```python
from build123d import *

# Parameters (mm, degrees)
F1_DEPTH = 11.0582
F2_SCALE = 0.3


with BuildPart() as f1:
    # F0 (on Front) → F1 (new body)
    with BuildSketch(Plane.XZ):
        Polygon((0.806323, 147.5619096), (-16.5301676, 29.8349162), (-49.993677, 60.879355), (-34.673032, 17.3364906), (-113.2920772, 8.063484), (-32.657161, -10.8857288), (-59.2666836, -42.736516), (-16.9333418, -25.8031742), (-2.54e-05, -147.5619096), (16.5301422, -24.9968258), (60.4761808, -42.3333418), (34.2698324, -10.0793804), (113.2920518, 8.4666582), (35.479355, 17.3364906), (49.9936262, 60.4761808), (16.9333164, 27.8190452), align=None)
    extrude(amount=F1_DEPTH)


with BuildPart() as f1_1:
    # F2: moved
    add(f1.part.scale(F2_SCALE).moved(Location((0.5644261, -7.74074, 103.29333672))))


with BuildPart() as f1_2:
    # F3: moved
    add(f1_1.part.moved(Location((59.91897, 0, -43.45396))))


solid = f1_2.part
```
Here's how the part is built. I have some questions about the finished solid (model axes, mm). A direction names the side the tool comes from. Give positions to 0.01 mm unless a question says otherwise; leave off trailing zeros. Loops run counter-clockwise (first coordinate to the right, second up) from the corner with the lowest first, then second, coordinate; pieces in that order, holes last. Notation, with made-up numbers: (55.5, 9) -> (94.5, 9) arc R12 cw to (94.5, 20) -> close; hole circle Ø1 at (43.25, 72.5). An arc over 180 degrees is marked (long way). Use one line per item in the form item = value. Start each with the question number.
1) Imagine slicing it at A-A (z = 74). Please give me the cut outline in (x, y), then the cut area to 3 significant figures.
2) Which directions (+Z, -Z, +X, -X, +Y, -Y) give clear straight access to the entire face, cutting with the end or side of a thin tool? Please do faces 5 (the face through (71.942, -9.376, 49.776)), 6 (the face through (74.75, -9.38, 51.91)), 7 (the face through (60, -7.741, 60)), 8 (the face through (38.45, -9.38, 63.67)), 9 (the face through (50.575, -9.376, 73.381)).
3) Imagine slicing it at B-B (x = 46.5). Please give me the cut outline in (y, z), then the cut area to 3 significant figures.
4) Imagine slicing it at C-C (y = -9.25). Please give me the cut outline in (x, z), then the cut area to 3 significant figures.
5) Imagine slicing it at D-D (x = 31.5). Please give me the cut outline in (y, z).
6) Thinking about a two-plate mould opening in X: for faces 1 (the face through (47.751, -9.376, 71.663)), 2 (the face through (48.96, -9.38, 49.52)), 3 (the face through (70.59, -9.38, 73.15)), 4 (the face through (82.96, -9.38, 63.69)), which applies, +X half, -X half, draft (parallel to the pull), parting line (faces both ways), or undercut?
7) Please list where these lines run through material, in increasing order: line 1 along X through (y, z) = (-10, 73); line 2 along X through (y, z) = (-8.3, 76.5); line 3 along Z through (x, y) = (77, -9.55).
Check values:
q1.outline = (46.93, -11.06) -> (49.91, -11.06) -> (49.91, -7.74) -> (46.93, -7.74) -> close; (56.29, -11.06) -> (64.78, -11.06) -> (64.78, -7.74) -> (56.29, -7.74) -> close; (71.45, -11.06) -> (74.14, -11.06) -> (74.14, -7.74) -> (71.45, -7.74) -> close
q1.area = 47.0 mm^2
q2.face_5 = -Z, +Y, -Y
q2.face_6 = +X, +Y, -Y
q2.face_7 = +Z, -Z, +X, -X, +Y
q2.face_8 = -X, +Y, -Y
q2.face_9 = +Z, +Y, -Y
q3.outline = (-11.06, 48.54) -> (-7.74, 48.54) -> (-7.74, 51.56) -> (-11.06, 51.56) -> close; (-11.06, 57.56) -> (-7.74, 57.56) -> (-7.74, 64.62) -> (-11.06, 64.62) -> close; (-11.06, 75.22) -> (-7.74, 75.22) -> (-7.74, 77.16) -> (-11.06, 77.16) -> close
q3.area = 39.9 mm^2
q4.outline = (26.5, 62.26) -> (50.69, 56.57) -> (42.7, 47.02) -> (55.4, 52.1) -> (60.48, 15.57) -> (65.44, 52.34) -> (78.63, 47.14) -> (70.76, 56.82) -> (94.47, 62.38) -> (71.13, 65.04) -> (75.48, 77.98) -> (65.56, 68.19) -> (60.73, 104.11) -> (55.52, 68.79) -> (45.49, 78.1) -> (50.08, 65.04) -> close
q4.area = 1,020 mm^2
q5.outline = (-11.06, 61.08) -> (-7.74, 61.08) -> (-7.74, 62.85) -> (-11.06, 62.85) -> close
q6.face_1 = -X half
q6.face_2 = undercut
q6.face_3 = undercut
q6.face_4 = +X half
q7.line_1 = 47.28 to 50.99, 56.14 to 64.91, 70.44 to 73.81
q7.line_2 = 46.05 to 47.21, 56.66 to 64.44, 73.98 to 74.98
q7.line_3 = 47.78 to 49.14, 58.28 to 64.37
